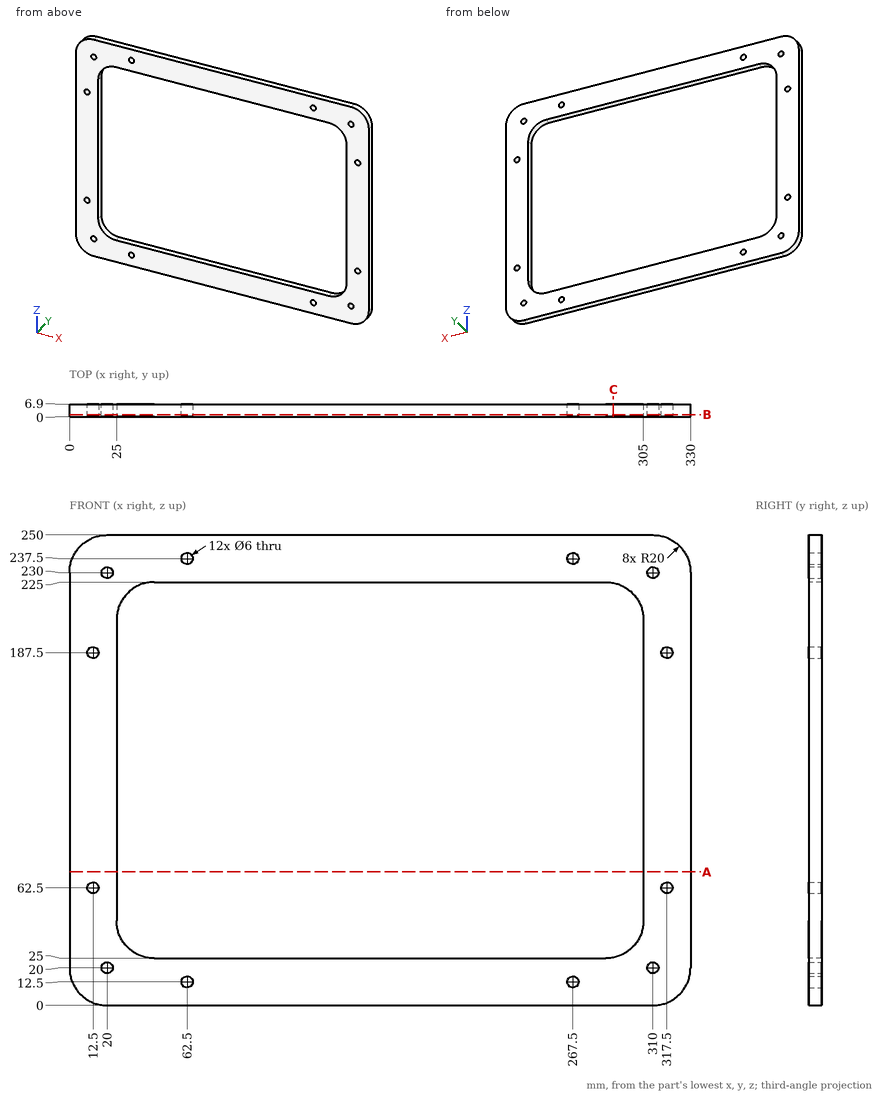
Geometry check sheet. Reference: drawing and pictorial views, mm from the part's lowest x, y, z. Round coordinates to 2 decimals unless told otherwise and drop trailing zeros. Write each loop counter-clockwise with the first axis right and the second up, starting at its lowest first coordinate (ties: lowest second). Pieces come first, ordered by that corner, then holes. Notation, with made-up numbers: (13.5, 52.25) -> (46.5, 52.25) arc R15 ccw to (46.5, 61.25) -> close; hole circle Ø11 at (-18.5, 7). An arc over 180 degrees is marked (long way). One line per question, with ' | ' between items. Start each with the question number.
1. Sectioned sample at A-A, the plane z = 71. Record the cut outline in (x, y), then the cut area to 3 significant figures.
2. Sectioned sample at C-C, the plane x = 289. Record the cut outline in (y, z), then the cut area to 3 significant figures.
3. Scan lines: line 1 along Z through (x, y) = (309.5, 4); line 2 along X through (y, z) = (1.75, 20); line 3 along X through (y, z) = (2.5, 62.5). Record each from-to range of solid material in increasing order. Write a range as from..to.
4. Depth check by flat-ended pin: pin 1 (7 mm diameter, centred on x = 310, z = 20, fed in from +Y). Enter the tip coordinate at first touch or a pass-through.
5. Sectioned sample at B-B, the plane y = 1.25. Count the separate pieces of the cut face and the enclosed holes in it, then the cut area to 3 significant figures.
Taken from the geometry:
1) outline: (0, 0) -> (25, 0) -> (25, 6.9) -> (0, 6.9) -> close; (305, 0) -> (330, 0) -> (330, 6.9) -> (305, 6.9) -> close | area: 345 mm^2
2) outline: (0, 0) -> (6.9, 0) -> (6.9, 25.4) -> (0, 25.4) -> close; (0, 224.6) -> (6.9, 224.6) -> (6.9, 250) -> (0, 250) -> close | area: 351 mm^2
3) line 1: z = 0..17.04, 22.96..227.04, 232.96..250 | line 2: x = 0..17, 23..307, 313..330 | line 3: x = 0..9.5, 15.5..25, 305..314.5, 320.5..330
4) pin 1: stops at y = 6.9
5) separate pieces: 1 | enclosed holes: 13 | area: 26,200 mm^2
